Design review of the part built by this model. Coordinates are the model's own, in mm. Face numbers are marked on the shaded views. A direction names the side the tool comes from. Coordinates: 2 decimals unless noted, no trailing zeros. Write each loop counter-clockwise with the first axis right and the second up, starting at its lowest first coordinate (ties: lowest second). Pieces come first, ordered by that corner, then holes.
Q1. Add section D-D, the plane x = 210. Give the boundary of the cut face in (y, z).
Q2. Add section A-A, the plane x = 120. Give the boundary of the cut face in (y, z).
Q3. Machinability: for the marked faces 1, 2, 3, 4 and 5, which of the approach directions +Z, -Z, +X, -X, +Y, -Y give a long, thin tool a straight path to every point of the face, cutting with its end or side? Answer none if there is none.
Q4. Add section C-C, the plane y = 83.5. Give the boundary of the cut face in (x, z), plus the area to 3 significant figures.
Q5. Add section B-B, the plane y = 15.5. Give the boundary of the cut face in (x, z).
Q6. To check wall thickness, follow probe 1 along X at (y, z) = (175.5, -158); probe 2 along Y at (x, z) = (210, -165.5); probe 3 along Z at (x, y) = (56.5, 180). State the ranges of each line that lie inside material, in increasing order.
Q7. Clearance check with flat-ended pins moving along their axes: pin 1 Ø5 at (y, z) = (118, -154.5) entering from -X; pin 2 Ø11 at (x, z) = (322.5, -156) entering from -Y; pin 3 Ø8 at (y, z) = (107.5, -195.5) entering from +X. State where each tip first meets the part, or that it passes through.
Q8. The part is to be moulded in two halves that separate along X. For the marked faces 6 and 7, say which applies: +X half, -X half, draft (parallel to the pull), parting line (faces both ways), or undercut.
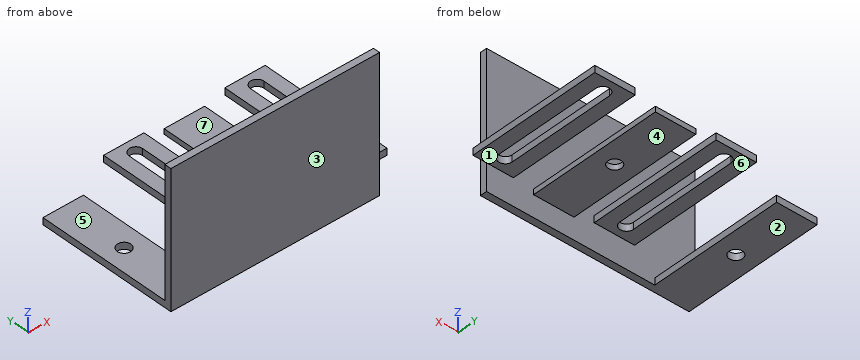
from build123d import *

# Parameters (mm, degrees)
SKETCH1_W           = 310
SKETCH1_H           = 200
BOSS_EXTRUDE1_DEPTH = 10
SKETCH2_W           = 60
SKETCH2_H           = 10
SKETCH2_H_2         = 7.912912389
BOSS_EXTRUDE2_DEPTH = 200
SKETCH3_R           = 10
CUT_EXTRUDE1_DEPTH  = 200


with BuildPart() as part:
    # Sketch1 → Boss-Extrude1 (new body)
    with BuildSketch(Plane(origin=(0, 0, 0), x_dir=(1, 0, 0), z_dir=(0, 1, 0))):
        with Locations((155, 100)):
            Rectangle(SKETCH1_W, SKETCH1_H)
    extrude(amount=BOSS_EXTRUDE1_DEPTH)

    # Sketch2 → Boss-Extrude2 (add)
    with BuildSketch(Plane(origin=(0, 10, 0), x_dir=(1, 0, 0), z_dir=(0, 1, 0))):
        with Locations((30, 195)):
            Rectangle(SKETCH2_W, SKETCH2_H)
        with Locations((120, 155)):
            Rectangle(SKETCH2_W, SKETCH2_H)
        with Locations((300, 155)):
            Rectangle(SKETCH2_W, SKETCH2_H)
        with Locations((210, 163.956456194)):
            Rectangle(SKETCH2_W, SKETCH2_H_2)
    extrude(amount=BOSS_EXTRUDE2_DEPTH)

    # Sketch3 → Cut-Extrude1 (cut)
    with BuildSketch(Plane.XY.offset(-150)):
        with Locations((30, 110)):
            Circle(SKETCH3_R)
        with Locations((210, 110)):
            Circle(SKETCH3_R)
        with BuildLine():
            Line((110, 190), (110, 30))
            ThreePointArc((110, 30), (120, 20), (130, 30))
            Line((130, 30), (130, 190))
            ThreePointArc((130, 190), (120, 200), (110, 190))
        make_face()
        with BuildLine():
            Line((290, 190), (290, 30))
            ThreePointArc((290, 30), (300, 20), (310, 30))
            Line((310, 30), (310, 190))
            ThreePointArc((310, 190), (300, 200), (290, 190))
        make_face()
    extrude(amount=-CUT_EXTRUDE1_DEPTH, mode=Mode.SUBTRACT)


solid = part.part
Here are the results:
1. outline: (0, -200) - (10, -200) - (10, -167.91) - (100, -167.91) - (100, -160) - (10, -160) - (10, 0) - (0, 0) - close; (120, -167.91) - (210, -167.91) - (210, -160) - (120, -160) - close
2. outline: (0, -200) - (10, -200) - (10, -160) - (20, -160) - (20, -150) - (10, -150) - (10, 0) - (0, 0) - close; (200, -160) - (210, -160) - (210, -150) - (200, -150) - close
3. face 1: -Z, +X, +Y
3. face 2: -Z, +X, -X, +Y, -Y
3. face 3: +Z, -Z, +X, -X, -Y
3. face 4: -Z, +X, -X, +Y
3. face 5: +Z, +X, -X, +Y
4. outline: (0, -200) - (60, -200) - (60, -190) - (0, -190) - close; (90, -160) - (110, -160) - (110, -150) - (90, -150) - close; (130, -160) - (150, -160) - (150, -150) - (130, -150) - close; (180, -167.91) - (240, -167.91) - (240, -160) - (180, -160) - close; (270, -160) - (290, -160) - (290, -150) - (270, -150) - close; (310, -160) - (330, -160) - (330, -150) - (310, -150) - close
4. area: 1,870 mm2
5. outline: (0, -200) - (60, -200) - (60, -190) - (0, -190) - close; (90, -160) - (150, -160) - (150, -150) - (90, -150) - close; (180, -167.91) - (240, -167.91) - (240, -160) - (180, -160) - close; (270, -160) - (330, -160) - (330, -150) - (270, -150) - close
6. probe 1: x = 90 to 110, 130 to 150, 270 to 290, 310 to 330
6. probe 2: y = 0 to 100, 120 to 210
6. probe 3: z = -200 to -190
7. pin 1: stops at x = 90
7. pin 2: stops at y = 10
7. pin 3: stops at x = 60
8. face 6: draft
8. face 7: undercut
